from build123d import *

# Parameters (mm, degrees)
F1_DEPTH = 60
F2_W     = 3.727922
F2_H     = 3
F3_DEPTH = 3


with BuildPart() as f1:
    # F0 (on Top) → F1 (new body)
    with BuildSketch(Plane.XY):
        Polygon((-59.501522, 25.738621), (-56.865483, 28.37466), (-56.865483, 32.102582), (-59.501522, 34.738621), (-63.229444, 34.738621), (-65.865483, 32.102582), (-65.865483, 28.37466), (-63.229444, 25.738621), align=None)
    extrude(amount=F1_DEPTH)

    # F2 (on face) → F3 (join)
    with BuildSketch(Plane(origin=(-65.865483, 0, 0), x_dir=(0, -1, 0), z_dir=(-1, 0, 0))):
        with Locations((-30.238621, 1.5)):
            Rectangle(F2_W, F2_H)
    extrude(amount=F3_DEPTH)


solid = f1.part
Read the model definition and answer for the solid it produces. Units are mm, in the model's axes. A direction names the side the tool comes from. Round coordinates to 2 decimals unless told otherwise and drop trailing zeros. Write each loop counter-clockwise with the first axis right and the second up, starting at its lowest first coordinate (ties: lowest second). Pieces come first, ordered by that corner, then holes. Notation, with made-up numbers: (83.5, 70) - (125.5, 70) arc R18 ccw to (125.5, 79) - close; hole circle Ø6 at (-35, 13.25). An arc over 180 degrees is marked (long way). Use a Markdown table: item, result.
(1) Which of the six approach directions +Z, -Z, +X, -X, +Y, -Y give full straight-line access (tool end or side, diameter ignored) to faces 1 (the flat face through (-65.865, 30, 31)), 2 (the flat face through (-61, 25.739, 30)), 3 (the flat face through (-67, 28.375, 1)), 4 (the flat face through (-68.865, 30, 2)), 5 (the flat face through (-67, 32.103, 1))?
Reported:
| item | result |
|---|---|
| face 1 | +Z, -X, +Y, -Y |
| face 2 | +Z, -Z, +X, -X, -Y |
| face 3 | +Z, -Z, -X, -Y |
| face 4 | +Z, -Z, -X, +Y, -Y |
| face 5 | +Z, -Z, -X, +Y |
(2) The part is cut by section C-C (x = -67.75). Write down the section's boundary in (y, z), then the cut area to 3 significant figures.
Reported:
| item | result |
|---|---|
| outline | (28.37, 0) - (32.1, 0) - (32.1, 3) - (28.37, 3) - close |
| area | 11.2 mm2 |
(3) Straight lines are drawn through the part: line 1 along Z through (x, y) = (-66.5, 30); line 2 along X through (y, z) = (32, 9.5); line 3 along Y through (x, z) = (-59, 50). For each, find the intervals that lie inside material, in ascending order. Write a range as [from, to].
Reported:
| item | result |
|---|---|
| line 1 | [0, 3] |
| line 2 | [-65.87, -56.87] |
| line 3 | [26.24, 34.24] |
(4) The part is cut by section B-B (y = 29). Write down the section's boundary in (x, z), then the cut area to 3 significant figures.
Reported:
| item | result |
|---|---|
| outline | (-68.87, 0) - (-56.87, 0) - (-56.87, 60) - (-65.87, 60) - (-65.87, 3) - (-68.87, 3) - close |
| area | 549 mm2 |
(5) The part is cut by section A-A (z = 42.5). Write down the section's boundary in (x, y).
Reported:
| item | result |
|---|---|
| outline | (-65.87, 28.37) - (-63.23, 25.74) - (-59.5, 25.74) - (-56.87, 28.37) - (-56.87, 32.1) - (-59.5, 34.74) - (-63.23, 34.74) - (-65.87, 32.1) - close |
(6) Each of these flat-tipped pins is pushed along its axis until it touches: pin 1 Ø1.9 at (y, z) = (30.5, 24.5) entering from -X; pin 2 Ø2.5 at (x, z) = (-68, 2) entering from -Y; pin 3 Ø1.5 at (x, z) = (-65, 51.5) entering from -Y. Where does it stop, or does it pass through?
Reported:
| item | result |
|---|---|
| pin 1 | x = -65.87 |
| pin 2 | y = 28.37 |
| pin 3 | y = 26.76 |
(7) The part is cut by section D-D (x = -58). Write down the section's boundary in (y, z).
Reported:
| item | result |
|---|---|
| outline | (27.24, 0) - (33.24, 0) - (33.24, 60) - (27.24, 60) - close |
